Check sheet for the modelled part. Datum: model origin and axes. Units: mm. A direction names the side the tool comes from. Round coordinates to 2 decimals unless told otherwise and drop trailing zeros. Write each loop counter-clockwise with the first axis right and the second up, starting at its lowest first coordinate (ties: lowest second). Pieces come first, ordered by that corner, then holes. Notation, with made-up numbers: M 10.25,21 L 58.25,21 A31 ccw 58.25,60 Z; hole C 28.5,67.25 d2. An arc over 180 degrees is marked long. Answer in a Markdown table with one row per item.
```python
from build123d import *

# Parameters (mm, degrees)
BOSS_EXTRUDE1_DEPTH   = 4
F_2_5MM_DOWEL_HOLE1_D = 2.5
CIRPATTERN2_COUNT     = 12
F_2_5MM_DOWEL_HOLE2_D = 2.5
CUT_EXTRUDE1_DEPTH    = 85.947042326


with BuildPart() as part:
    # Sketch1 → Boss-Extrude1 (new body)
    with BuildSketch(Plane(origin=(0, 0, 0), x_dir=(1, 0, 0), z_dir=(0, 1, 0))):
        Polygon((0, 60), (-30, 51.961524227), (-51.961524227, 30), (-60, 0), (-51.961524227, -30), (-30, -51.961524227), (0, -60), (30, -51.961524227), (51.961524227, -30), (60, 0), (51.961524227, 30), (30, 51.961524227), align=None)
    extrude(amount=BOSS_EXTRUDE1_DEPTH)

    # 2.5mm Dowel Hole1 (through all)
    with Locations(Plane(origin=(0, 4, 0), x_dir=(1, 0, 0), z_dir=(0, 1, 0))):
        with Locations((-46.991169754, 20.82821885), (-20.82821885, 46.991169754)):
            f_2_5mm_dowel_hole1 = Hole(F_2_5MM_DOWEL_HOLE1_D / 2)

    # CirPattern2: 2.5mm Dowel Hole1 ×12 about axis
    cirpattern2_axis = Axis((0, 0, 0), (0, 1, 0))
    for i in range(1, CIRPATTERN2_COUNT):
        add(f_2_5mm_dowel_hole1.rotate(cirpattern2_axis, i * 360 / CIRPATTERN2_COUNT), mode=Mode.SUBTRACT)

    # 2.5mm Dowel Hole2 (through all)
    with Locations(Plane(origin=(0, 4, 0), x_dir=(1, 0, 0), z_dir=(0, 1, 0))):
        with Locations((-45.254833996, 8.485281374), (-8.485281374, 45.254833996), (45.961940777, -7.778174593), (7.778174593, -45.961940777)):
            Hole(F_2_5MM_DOWEL_HOLE2_D / 2)

    # Sketch10 → Cut-Extrude1 (cut, through all)
    with BuildSketch(Plane(origin=(0, 4, 0), x_dir=(1, 0, 0), z_dir=(0, 1, 0))):
        Polygon((0, 42), (-21, 36.373066959), (-36.373066959, 21), (-42, 0), (-36.373066959, -21), (-21, -36.373066959), (0, -42), (21, -36.373066959), (36.373066959, -21), (42, 0), (36.373066959, 21), (21, 36.373066959), align=None)
    extrude(amount=-CUT_EXTRUDE1_DEPTH, mode=Mode.SUBTRACT)


solid = part.part
```
1. Section check A-A, the plane z = 14.5. Record the cut outline in (x, y), and give its area (3 significant figures).
Found:
| item | result |
|---|---|
| outline | M -56.11,0 L -38.11,0 L -38.11,4 L -56.11,4 Z; M 38.11,0 L 56.11,0 L 56.11,4 L 38.11,4 Z |
| area | 144 mm2 |
2. Section check C-C, the plane y = 2.4. Count the separate pieces of the cut face and the enclosed holes in it, and give its area (3 significant figures).
Found:
| item | result |
|---|---|
| separate pieces | 1 |
| enclosed holes | 29 |
| area | 5,370 mm2 |
3. Section check B-B, the plane x = -12.5. Record the cut outline in (y, z).
Found:
| item | result |
|---|---|
| outline | M 0,-56.65 L 4,-56.65 L 4,-38.65 L 0,-38.65 Z; M 0,38.65 L 4,38.65 L 4,56.65 L 0,56.65 Z |
4. Scan lines: L1, parallel to Z at x = -51.5, y = 0.2; L2, parallel to X at y = 3.8, z = 31; L3, parallel to Z at x = 29.5, y = 2.5. Record each from-to range of solid material in increasing order.
Found:
| item | result |
|---|---|
| L1 | z = -30.46 to -6.65, -4.27 to 4.27, 6.65 to 30.46 |
| L2 | x = -50.96 to -42.56, -40.51 to -26.37, 26.37 to 40.51, 42.56 to 50.96 |
| L3 | z = -52.1 to -42.51, -40.56 to -27.87, 27.87 to 40.56, 42.51 to 52.1 |
5. Go/stop test with flat-tipped pins: pin 1 (1 mm diameter, centred on x = 2, y = 1, fed in from +Z); pin 2 (2 mm diameter, centred on x = -51.11, z = -5.46, fed in from -Y); pin 3 (3 mm diameter, centred on x = -8.49, z = -45.25, fed in from -Y); pin 4 (1.5 mm diameter, centred on x = 46, y = 2, fed in from +Z). Record where each tip stops, or that it passes through.
Found:
| item | result |
|---|---|
| pin 1 | stops at z = 59.6 |
| pin 2 | passes through |
| pin 3 | stops at y = 0 |
| pin 4 | stops at z = 36.71 |
6. Draft check along Z on faces 1 (the face through (28.794, 2.028, -28.579)), 2 (the face through (10.353, 2.028, 39.226)), 3 (the face through (39, 0, 12)), 4 (the face through (-55.924, 1.972, -15.21)). Enter one of: +Z half, -Z half, draft (parallel to the pull), parting line (faces both ways), or undercut.
Found:
| item | result |
|---|---|
| face 1 | undercut |
| face 2 | undercut |
| face 3 | draft |
| face 4 | -Z half |
7. Access from +Z, -Z, +X, -X, +Y, -Y to the whole of each face (thin tool, end or side, straight path). Record for faces 5 (the face through (-39.226, 2.028, 10.353)), 6 (the face through (-41.13, 1.97, 40.83)).
Found:
| item | result |
|---|---|
| face 5 | +Y, -Y |
| face 6 | +Z, -X, +Y, -Y |
